Check sheet for the modelled part. Datum: model origin and axes. Units: mm. Face numbers are marked on the shaded views. A direction names the side the tool comes from. Round coordinates to 2 decimals unless told otherwise and drop trailing zeros. Order: outer loops, then holes, each group sorted by start corner. A loop starts at its lowest first (then second) coordinate and runs counter-clockwise, first axis right, second up.
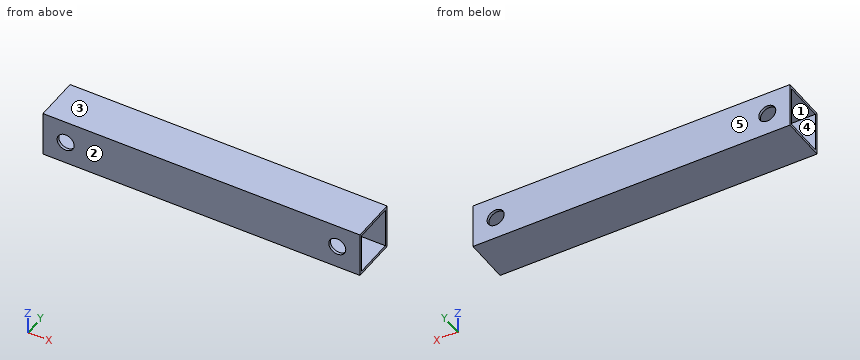
```python
from build123d import *

# Parameters (mm, degrees)
SKETCH1_W           = 25.4
SKETCH1_H           = 25.4
SKETCH1_W_2         = 22.225
SKETCH1_H_2         = 22.225
BOSS_EXTRUDE1_DEPTH = 177.8
SKETCH2_R           = 4.7625
CUT_EXTRUDE1_DEPTH  = 181.05357536


with BuildPart() as part:
    # Sketch1 → Boss-Extrude1 (new body)
    with BuildSketch(Plane(origin=(0, 0, 0), x_dir=(0, 0, -1), z_dir=(1, 0, 0))):
        Rectangle(SKETCH1_W, SKETCH1_H)
        Rectangle(SKETCH1_W_2, SKETCH1_H_2, mode=Mode.SUBTRACT)
    extrude(amount=BOSS_EXTRUDE1_DEPTH)

    # Sketch2 → Cut-Extrude1 (cut, through all)
    with BuildSketch(Plane(origin=(0, 12.7, 0), x_dir=(1, 0, 0), z_dir=(0, 1, 0))):
        with Locations(Location((12.7, 0, 0), (0, 0, 270))):
            Circle(SKETCH2_R)
        with Locations(Location((165.1, 0, 0), (0, 0, 270))):
            Circle(SKETCH2_R)
    extrude(amount=-CUT_EXTRUDE1_DEPTH, mode=Mode.SUBTRACT)


solid = part.part
```
Item 1: Release check for a two-part mould opening along Y. For the marked faces 1, 2 and 3 record: released by +Y, released by -Y, zero draft, split by the parting line, or undercut.
Answer:
face 1: undercut
face 2: released by -Y
face 3: zero draft
Item 2: Scan lines: line 1 along X through (y, z) = (11.7, 0); line 2 along Y through (x, z) = (21, -7.5). Record each from-to range of solid material in increasing order.
Answer:
line 1: x = 0 to 7.94, 17.46 to 160.34, 169.86 to 177.8
line 2: y = -12.7 to -11.11, 11.11 to 12.7
Item 3: Go/stop test with a flat-tipped pin: P1, Ø5.5, axis at x = 165.1, z = 0, coming from the -Y side. Record where the tip stops, or that it passes through.
Answer:
P1: passes through
Item 4: Sectioned sample at D-D (x = 147.5). Record the cut outline in (y, z), and give its area (3 significant figures).
Answer:
outline: (-12.7, -12.7) - (12.7, -12.7) - (12.7, 12.7) - (-12.7, 12.7) - close; hole (-11.11, -11.11) - (11.11, -11.11) - (11.11, 11.11) - (-11.11, 11.11) - close
area: 151 mm2
Item 5: Sectioned sample at A-A (x = 12.7). Record the cut outline in (y, z), and give its area (3 significant figures).
Answer:
outline: (-12.7, -12.7) - (12.7, -12.7) - (12.7, -4.76) - (11.11, -4.76) - (11.11, -11.11) - (-11.11, -11.11) - (-11.11, -4.76) - (-12.7, -4.76) - close; (-12.7, 4.76) - (-11.11, 4.76) - (-11.11, 11.11) - (11.11, 11.11) - (11.11, 4.76) - (12.7, 4.76) - (12.7, 12.7) - (-12.7, 12.7) - close
area: 121 mm2
Item 6: Access from +Z, -Z, +X, -X, +Y, -Y to the whole of each face (thin tool, end or side, straight path). Record for the marked faces 4 and 5.
Answer:
face 4: +X, -X
face 5: +Z, -Z, +X, -X, +Y
Item 7: Sectioned sample at C-C (z = 0). Record the cut outline in (x, y), and give its area (3 significant figures).
Answer:
outline: (0, -12.7) - (7.94, -12.7) - (7.94, -11.11) - (0, -11.11) - close; (0, 11.11) - (7.94, 11.11) - (7.94, 12.7) - (0, 12.7) - close; (17.46, -12.7) - (160.34, -12.7) - (160.34, -11.11) - (17.46, -11.11) - close; (17.46, 11.11) - (160.34, 11.11) - (160.34, 12.7) - (17.46, 12.7) - close; (169.86, -12.7) - (177.8, -12.7) - (177.8, -11.11) - (169.86, -11.11) - close; (169.86, 11.11) - (177.8, 11.11) - (177.8, 12.7) - (169.86, 12.7) - close
area: 504 mm2
Item 8: Sectioned sample at B-B (y = -6.5). Record the cut outline in (x, z), and give its area (3 significant figures).
Answer:
outline: (0, -12.7) - (177.8, -12.7) - (177.8, -11.11) - (0, -11.11) - close; (0, 11.11) - (177.8, 11.11) - (177.8, 12.7) - (0, 12.7) - close
area: 565 mm2
